```python
from build123d import *

# Parameters (mm, degrees)
F0_R     = 7.62
F1_DEPTH = 1.27
F3_DEPTH = 1.27
F5_DEPTH = 1.27


with BuildPart() as f1:
    # F0 (on Front) → F1 (new body, symmetric)
    with BuildSketch(Plane.XZ):
        Circle(F0_R)
    extrude(amount=F1_DEPTH, both=True)

    # F2 (on face) → F3 (cut)
    with BuildSketch(Plane.XZ.offset(1.27)):
        with BuildLine():
            Line((7.6050439154, -0.4771865936), (0.4771865936, -7.6050439154))
            ThreePointArc((0.4771865936, -7.6050439154), (1.6514714828, -7.438887144), (2.7857510969, -7.0925306362))
            Line((2.7857510969, -7.0925306362), (7.0925306362, -2.7857510969))
            ThreePointArc((7.0925306362, -2.7857510969), (7.438887144, -1.6514714828), (7.6050439154, -0.4771865936))
        make_face()
        with BuildLine():
            Line((7.1432154673, 2.6530874068), (-2.6530874068, -7.1432154673))
            ThreePointArc((-2.6530874068, -7.1432154673), (-1.9523045555, -7.3656572635), (-1.2333458364, -7.5195251212))
            Line((-1.2333458364, -7.5195251212), (7.5195251212, 1.2333458364))
            ThreePointArc((7.5195251212, 1.2333458364), (7.3656572635, 1.9523045555), (7.1432154673, 2.6530874068))
        make_face()
        with BuildLine():
            Line((5.8184250178, 4.9203994057), (-4.9203994057, -5.8184250178))
            ThreePointArc((-4.9203994057, -5.8184250178), (-4.410994208, -6.2134958032), (-3.8700189421, -6.5640957784))
            Line((-3.8700189421, -6.5640957784), (6.5640957784, 3.8700189421))
            ThreePointArc((6.5640957784, 3.8700189421), (6.2134958032, 4.410994208), (5.8184250178, 4.9203994057))
        make_face()
        with BuildLine():
            Line((3.8700189421, 6.5640957784), (-6.5640957784, -3.8700189421))
            ThreePointArc((-6.5640957784, -3.8700189421), (-6.2134958032, -4.410994208), (-5.8184250178, -4.9203994057))
            Line((-5.8184250178, -4.9203994057), (4.9203994057, 5.8184250178))
            ThreePointArc((4.9203994057, 5.8184250178), (4.410994208, 6.2134958032), (3.8700189421, 6.5640957784))
        make_face()
        with BuildLine():
            Line((1.2333458364, 7.5195251212), (-7.5195251212, -1.2333458364))
            ThreePointArc((-7.5195251212, -1.2333458364), (-7.3656572635, -1.9523045555), (-7.1432154673, -2.6530874068))
            Line((-7.1432154673, -2.6530874068), (2.6530874068, 7.1432154673))
            ThreePointArc((2.6530874068, 7.1432154673), (1.9523045555, 7.3656572635), (1.2333458364, 7.5195251212))
        make_face()
        with BuildLine():
            Line((-2.7857510969, 7.0925306362), (-7.0925306362, 2.7857510969))
            ThreePointArc((-7.0925306362, 2.7857510969), (-7.438887144, 1.6514714828), (-7.6050439154, 0.4771865936))
            Line((-7.6050439154, 0.4771865936), (-0.4771865936, 7.6050439154))
            ThreePointArc((-0.4771865936, 7.6050439154), (-1.6514714828, 7.438887144), (-2.7857510969, 7.0925306362))
        make_face()
    extrude(amount=-F3_DEPTH, mode=Mode.SUBTRACT)

    # F4 (on face) → F5 (cut)
    with BuildSketch(Plane(origin=(0, 1.27, 0), x_dir=(-1, 0, 0), z_dir=(0, 1, 0))):
        with BuildLine():
            ThreePointArc((-7.0925306362, 2.7857510969), (-7.438887144, 1.6514714828), (-7.6050439154, 0.4771865936))
            Line((-7.6050439154, 0.4771865936), (-0.4771865936, 7.6050439154))
            ThreePointArc((-0.4771865936, 7.6050439154), (-1.6514714828, 7.438887144), (-2.7857510969, 7.0925306362))
            Line((-2.7857510969, 7.0925306362), (-7.0925306362, 2.7857510969))
        make_face()
        with BuildLine():
            ThreePointArc((-7.5195251212, -1.2333458364), (-7.3656572635, -1.9523045555), (-7.1432154673, -2.6530874068))
            Line((-7.1432154673, -2.6530874068), (2.6530874068, 7.1432154673))
            ThreePointArc((2.6530874068, 7.1432154673), (1.9523045555, 7.3656572635), (1.2333458364, 7.5195251212))
            Line((1.2333458364, 7.5195251212), (-7.5195251212, -1.2333458364))
        make_face()
        with BuildLine():
            ThreePointArc((-6.5640957784, -3.8700189421), (-6.2134958032, -4.410994208), (-5.8184250178, -4.9203994057))
            Line((-5.8184250178, -4.9203994057), (4.9203994057, 5.8184250178))
            ThreePointArc((4.9203994057, 5.8184250178), (4.410994208, 6.2134958032), (3.8700189421, 6.5640957784))
            Line((3.8700189421, 6.5640957784), (-6.5640957784, -3.8700189421))
        make_face()
        with BuildLine():
            ThreePointArc((-4.9203994057, -5.8184250178), (-4.410994208, -6.2134958032), (-3.8700189421, -6.5640957784))
            Line((-3.8700189421, -6.5640957784), (6.5640957784, 3.8700189421))
            ThreePointArc((6.5640957784, 3.8700189421), (6.2134958032, 4.410994208), (5.8184250178, 4.9203994057))
            Line((5.8184250178, 4.9203994057), (-4.9203994057, -5.8184250178))
        make_face()
        with BuildLine():
            ThreePointArc((-2.6530874068, -7.1432154673), (-1.9523045555, -7.3656572635), (-1.2333458364, -7.5195251212))
            Line((-1.2333458364, -7.5195251212), (7.5195251212, 1.2333458364))
            ThreePointArc((7.5195251212, 1.2333458364), (7.3656572635, 1.9523045555), (7.1432154673, 2.6530874068))
            Line((7.1432154673, 2.6530874068), (-2.6530874068, -7.1432154673))
        make_face()
        with BuildLine():
            Line((2.7857510969, -7.0925306362), (7.0925306362, -2.7857510969))
            ThreePointArc((7.0925306362, -2.7857510969), (7.438887144, -1.6514714828), (7.6050439154, -0.4771865936))
            Line((7.6050439154, -0.4771865936), (0.4771865936, -7.6050439154))
            ThreePointArc((0.4771865936, -7.6050439154), (1.6514714828, -7.438887144), (2.7857510969, -7.0925306362))
        make_face()
    extrude(amount=-F5_DEPTH, mode=Mode.SUBTRACT)

    # F6 (on Top) → F7 (revolve, cut)
    with BuildSketch(Plane.XY):
        Polygon((-5.715, -1.27), (-7.62, 0), (-7.62, -1.27), align=None)
    revolve(axis=Axis((0, -1.3864838984, 0), (0, -1, 0)), mode=Mode.SUBTRACT)


solid = f1.part
```
CAD build for the part. Positions are in the model's coordinates, mm. A direction names the side the tool comes from. Round coordinates to 2 decimals unless told otherwise and drop trailing zeros. Order: outer loops, then holes, each group sorted by start corner. A loop starts at its lowest first (then second) coordinate and runs counter-clockwise, first axis right, second up. Notation, with made-up numbers: (78.5, 37.25) - (125.5, 37.25) arc R30 cw to (125.5, 61.25) - close; hole circle Ø5 at (-11, -37). An arc over 180 degrees is marked (long way). Answer as CSV lines item,"result". Start each with the question number.
1. Saw through at A-A, the plane y = 0.3. Write the cut outline in (x, z), and give its area (3 significant figures).
2. Pin check, flat tips, straight feed: pin 1 (0.5 mm diameter, centred on x = -0.5, z = 1, fed in from -Y); pin 2 (1.5 mm diameter, centred on x = 2.5, y = 1, fed in from -Z); pin 3 (0.5 mm diameter, centred on x = 4.5, z = -3, fed in from +Y). Stop position of each tip, or through.
3. Saw through at B-B, the plane y = -0.65. Write the cut outline in (x, z) (3 decimals), and give its area (3 significant figures).
4. Saw through at C-C, the plane x = 2. Count the separate pieces of the cut face and the enclosed holes in it, and give its area (3 significant figures).
5. Pull direction X, two halves, no side cores. Call faces 1 (the face through (5.106, -0.238, -5.165)), 2 (the face through (1.274, 0.644, 1.42)), 3 (the face through (-6.2, -0.6, -2.6)), 4 (the face through (-1, 0, 5)): +X half, -X half, draft (parallel to the pull), parting line (faces both ways), or undercut.
6. Drill centre lines: L1, parallel to X at y = 0.35, z = -2; L2, parallel to X at y = -0.2, z = -1.5; L3, parallel to Z at x = -2.75, y = 0.5. Where is each one in solid material? Low to high. Write a range as [from, to].
7. Tool access for faces 5 (the face through (-7.61, 0.63, 0.39)), 6 (the face through (-4.5, 0, 2.7)), 7 (the face through (4.09, -0.5, -3.99)): list every direction of +Z, -Z, +X, -X, +Y, -Y with a clear straight run to the whole face (end or side of a thin tool).
Model answer:
1,outline,"(-7.61, -0.48) - (-0.48, -7.61) arc R7.62 ccw to (1.23, -7.52) - (-7.52, 1.23) arc R7.62 ccw to start; (-7.14, 2.65) - (2.65, -7.14) arc R7.62 ccw to (3.87, -6.56) - (-6.56, 3.87) arc R7.62 ccw to start; (-7.09, -2.79) arc R7.62 ccw to (-2.79, -7.09) - close; (-5.82, 4.92) - (4.92, -5.82) arc R7.62 ccw to (5.82, -4.92) - (-4.92, 5.82) arc R7.62 ccw to start; (-3.87, 6.56) - (6.56, -3.87) arc R7.62 ccw to (7.14, -2.65) - (-2.65, 7.14) arc R7.62 ccw to start; (-1.23, 7.52) - (7.52, -1.23) arc R7.62 ccw to (7.61, 0.48) - (0.48, 7.61) arc R7.62 ccw to start; (2.79, 7.09) - (7.09, 2.79) arc R7.62 ccw to start"
1,area,"89.7 mm²"
2,pin 1,"stops at y = 0"
2,pin 2,"stops at z = -7.14"
2,pin 3,"stops at y = 0"
3,outline,"(-6.636, -0.35) - (0.35, 6.636) arc R6.645 ccw to (-1.644, 6.438) - (-6.438, 1.644) arc R6.645 ccw to start; (-6.373, -1.883) arc R6.645 ccw to (-5.849, -3.154) - (3.154, 5.849) arc R6.645 ccw to (1.883, 6.373) - close; (-5.126, -4.228) arc R6.645 ccw to (-4.228, -5.126) - (5.126, 4.228) arc R6.645 ccw to (4.228, 5.126) - close; (-3.154, -5.849) arc R6.645 ccw to (-1.883, -6.373) - (6.373, 1.883) arc R6.645 ccw to (5.849, 3.154) - close; (-0.35, -6.636) arc R6.645 ccw to (1.644, -6.438) - (6.438, -1.644) arc R6.645 ccw to (6.636, 0.35) - close"
3,area,"69.5 mm²"
4,separate pieces,"4"
4,enclosed holes,"0"
4,area,"17.7 mm²"
5,face 1,"+X half"
5,face 2,"undercut"
5,face 3,"-X half"
5,face 4,"undercut"
6,L1,"x = [-6.08, -4.29], [-2.49, -0.69], [1.1, 2.9], [4.69, 6.49]"
6,L2,"x = [-5.99, -4.19], [-2.4, -0.6], [1.19, 2.99], [4.79, 6.58]"
6,L3,"z = [-5.33, -3.54], [-1.74, 0.06], [1.85, 3.65], [5.44, 7.11]"
7,face 5,"-X, +Y, -Y"
7,face 6,"+Y"
7,face 7,"-Y"
